Verification items for the finished model (mm, model axes). Face numbers are marked on the shaded views. A direction names the side the tool comes from. Round coordinates to 2 decimals unless told otherwise and drop trailing zeros. Write each loop counter-clockwise with the first axis right and the second up, starting at its lowest first coordinate (ties: lowest second). Pieces come first, ordered by that corner, then holes. Notation, with made-up numbers: (-18.75, 55) -> (26.25, 55) arc R13 ccw to (26.25, 69) -> close; hole circle Ø9 at (44, -15). An arc over 180 degrees is marked (long way). Answer as a JSON object with one key per item and string values. Group by question number.
(1) Sectioned sample at B-B on x = 99. Record the cut outline in (y, z).
(2) Scan lines: L1, parallel to X at y = -124, z = 6; L2, parallel to X at y = 115.5, z = 27; L3, parallel to Y at x = -75, z = 2 (3 decimals). Record each from-to range of solid material in increasing order. Write a range as from..to.
(3) Set-up check for the marked faces 1, 2, 3, 4 and 5: record each of +Z, -Z, +X, -X, +Y, -Y from which the full face is reachable in a straight line by a thin tool's end or side.
(4) Sectioned sample at A-A on y = 70.5. Record the cut outline in (x, z) (3 decimals), and give its area (3 significant figures).
(5) Gauge pin test, flat ends, axial feed: pin 1 Ø1.5 at (x, z) = (-59, 37.5) entering from -Y; pin 2 Ø11.5 at (x, z) = (-100, 17.5) entering from +Y; pin 3 Ø2 at (y, z) = (-42, 13.5) entering from +X. Record the tip position at first contact, or that the pin passes through.
(6) Draft check along X on the marked faces 6, 7 and 8. Enter one of: released by +X, released by -X, zero draft, split by the parting line, or undercut.
```python
from build123d import *

# Parameters (mm, degrees)
F0_W     = 48.542209
F0_H     = 20.6375
F0_W_2   = 20.6375
F0_H_2   = 48.542209
F1_DEPTH = 50.8


with BuildPart() as f1:
    # F0 (on Top) → F1 (new body)
    with BuildSketch(Plane.XY):
        Polygon((0, -20.6375), (0, 0), (-20.6375, 0), (-20.6375, -146.704241), (-20.6375, -150.996204), (0, -150.996204), (0, -144.4625), (0, -123.825), (0, -103.1875), (0, -82.55), (0, -61.9125), (0, -41.275), align=None)
        Polygon((20.6375, 0), (0, 0), (0, -20.6375), (146.704241, -20.6375), (150.996204, -20.6375), (150.996204, 0), (144.4625, 0), (123.825, 0), (103.1875, 0), (82.55, 0), (61.9125, 0), (41.275, 0), align=None)
        Polygon((0, 20.6375), (0, 0), (20.6375, 0), (20.6375, 146.704241), (20.6375, 150.996204), (0, 150.996204), (0, 144.4625), (0, 123.825), (0, 103.1875), (0, 82.55), (0, 61.9125), (0, 41.275), align=None)
        Polygon((-20.6375, 0), (0, 0), (0, 20.6375), (-146.704241, 20.6375), (-150.996204, 20.6375), (-150.996204, 0), (-144.4625, 0), (-123.825, 0), (-103.1875, 0), (-82.55, 0), (-61.9125, 0), (-41.275, 0), align=None)
        Polygon((-20.6375, -146.704241), (-20.6375, 0), (-41.275, 0), (-41.275, -139.257324), (-41.275, -146.704241), align=None)
        Polygon((146.704241, -20.6375), (0, -20.6375), (0, -41.275), (139.257324, -41.275), (146.704241, -41.275), align=None)
        Polygon((20.6375, 146.704241), (20.6375, 0), (41.275, 0), (41.275, 139.257324), (41.275, 146.704241), align=None)
        Polygon((-146.704241, 20.6375), (0, 20.6375), (0, 41.275), (-139.257324, 41.275), (-146.704241, 41.275), align=None)
        Polygon((-41.275, -139.257324), (-41.275, 0), (-61.9125, 0), (-61.9125, -128.10643), (-61.9125, -139.257324), align=None)
        Polygon((139.257324, -41.275), (0, -41.275), (0, -61.9125), (128.10643, -61.9125), (139.257324, -61.9125), align=None)
        Polygon((41.275, 139.257324), (41.275, 0), (61.9125, 0), (61.9125, 128.10643), (61.9125, 139.257324), align=None)
        Polygon((-139.257324, 41.275), (0, 41.275), (0, 61.9125), (-128.10643, 61.9125), (-139.257324, 61.9125), align=None)
        Polygon((-61.9125, -128.10643), (-61.9125, 0), (-82.55, 0), (-82.55, -112.152128), (-82.55, -128.10643), align=None)
        Polygon((128.10643, -61.9125), (0, -61.9125), (0, -82.55), (112.152128, -82.55), (128.10643, -82.55), align=None)
        Polygon((61.9125, 128.10643), (61.9125, 0), (82.55, 0), (82.55, 112.152128), (82.55, 128.10643), align=None)
        Polygon((-128.10643, 61.9125), (0, 61.9125), (0, 82.55), (-112.152128, 82.55), (-128.10643, 82.55), align=None)
        Polygon((-82.55, -112.152128), (-82.55, 0), (-103.1875, 0), (-103.1875, -88.843285), (-103.1875, -112.152128), align=None)
        Polygon((112.152128, -82.55), (0, -82.55), (0, -103.1875), (88.843285, -103.1875), (112.152128, -103.1875), align=None)
        Polygon((82.55, 112.152128), (82.55, 0), (103.1875, 0), (103.1875, 88.843285), (103.1875, 112.152128), align=None)
        Polygon((-112.152128, 82.55), (0, 82.55), (0, 103.1875), (-88.843285, 103.1875), (-112.152128, 103.1875), align=None)
        with Locations((24.271104, -134.14375)):
            Rectangle(F0_W, F0_H)
        Polygon((-103.1875, -88.843285), (-103.1875, 0), (-123.825, 0), (-123.825, -48.542209), (-123.825, -88.843285), align=None)
        Polygon((88.843285, -103.1875), (0, -103.1875), (0, -123.825), (48.542209, -123.825), (88.843285, -123.825), align=None)
        with Locations((134.14375, 24.271104)):
            Rectangle(F0_W_2, F0_H_2)
        Polygon((103.1875, 88.843285), (103.1875, 0), (123.825, 0), (123.825, 48.542209), (123.825, 88.843285), align=None)
        with Locations((-24.271104, 134.14375)):
            Rectangle(F0_W, F0_H)
        Polygon((-88.843285, 103.1875), (0, 103.1875), (0, 123.825), (-48.542209, 123.825), (-88.843285, 123.825), align=None)
        with Locations((-134.14375, -24.271104)):
            Rectangle(F0_W_2, F0_H_2)
    extrude(amount=F1_DEPTH)


solid = f1.part
```
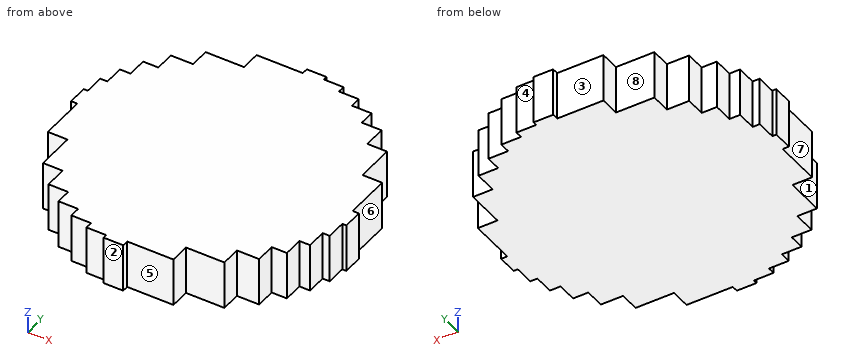
Computed values:
{
 "1": {"outline": "(-103.19, 0) -> (112.15, 0) -> (112.15, 50.8) -> (-103.19, 50.8) -> close"},
 "2": {"L1": "-82.55..48.54", "L2": "-88.84..82.55", "L3": "-128.106..123.825"},
 "3": {"face 1": "+Z, -Z, -X, -Y", "face 2": "+Z, -Z, +X, -X, -Y", "face 3": "+Z, -Z, -X, +Y", "face 4": "+Z, -Z, +X, +Y", "face 5": "+Z, -Z, +X, -Y"},
 "4": {"outline": "(-128.106, 0) -> (123.825, 0) -> (123.825, 50.8) -> (-128.106, 50.8) -> close", "area": "12,800 mm2"},
 "5": {"pin 1": "y = -139.26", "pin 2": "y = 103.19", "pin 3": "x = 146.7"},
 "6": {"face 6": "released by +X", "face 7": "released by -X", "face 8": "zero draft"}
}
